from build123d import *

# Parameters (mm, degrees)
SKETCH_W             = 65
SKETCH_H             = 30
SKETCH_R             = 7.6
PAD_DEPTH            = 22.5
SKETCH001_R          = 1.6
POCKET_DEPTH         = 12.001
POCKET_DEPTH_BACK    = -18.001
POCKET001_DEPTH      = 7
POCKET002_DEPTH      = 7
SKETCH004_R          = 5.1
POCKET003_DEPTH      = 8.5
SKETCH005_R          = 1.6
POCKET004_DEPTH      = 22.501
POCKET004_DEPTH_BACK = -22.501


with BuildPart() as part:
    # Sketch → Pad (new body, symmetric)
    with BuildSketch(Plane.XZ):
        with Locations((0, 3)):
            Rectangle(SKETCH_W, SKETCH_H)
        with Locations((-22.5, 0)):
            Circle(SKETCH_R, mode=Mode.SUBTRACT)
        with Locations((22.5, 0)):
            Circle(SKETCH_R, mode=Mode.SUBTRACT)
    extrude(amount=PAD_DEPTH, both=True)

    # Sketch001 → Pocket (cut, two sides)
    with BuildSketch(Plane.XY) as pocket_sk:
        with Locations((-12.5, 17.5)):
            Circle(SKETCH001_R)
        with Locations((12.5, 17.5)):
            Circle(SKETCH001_R)
        Circle(SKETCH001_R)
        with Locations((-12.5, -17.5)):
            Circle(SKETCH001_R)
        with Locations((12.5, -17.5)):
            Circle(SKETCH001_R)
        with Locations((0, 17.5)):
            Circle(SKETCH001_R)
        with Locations((0, -17.5)):
            Circle(SKETCH001_R)
    extrude(amount=-POCKET_DEPTH, mode=Mode.SUBTRACT)
    extrude(pocket_sk.sketch, amount=-POCKET_DEPTH_BACK, mode=Mode.SUBTRACT)

    # Sketch002 (on DatumPlane) → Pocket001 (cut)
    with BuildSketch(Plane.YZ.offset(2)):
        with BuildLine():
            ThreePointArc((-7, -1.25), (-3.464466, 0.214466), (-2, 3.75))
            Line((-2, 18), (-2, 3.75))
            Line((-14, 18), (-2, 18))
            Line((-14, 1.25), (-14, 18))
            Line((-22.5, 1.25), (-14, 1.25))
            Line((-22.5, -1.25), (-22.5, 1.25))
            Line((-7, -1.25), (-22.5, -1.25))
        make_face()
        with BuildLine():
            ThreePointArc((2, 3.75), (3.464466, 0.214466), (7, -1.25))
            Line((22.5, -1.25), (7, -1.25))
            Line((22.5, 1.25), (22.5, -1.25))
            Line((14, 1.25), (22.5, 1.25))
            Line((14, 18), (14, 1.25))
            Line((2, 18), (14, 18))
            Line((2, 3.75), (2, 18))
        make_face()
    extrude(amount=POCKET001_DEPTH, mode=Mode.SUBTRACT)

    # Sketch003 (on DatumPlane) → Pocket002 (cut)
    with BuildSketch(Plane.YZ.offset(-2)):
        with BuildLine():
            Line((-7, -1.25), (-22.5, -1.25))
            Line((-22.5, -1.25), (-22.5, 1.25))
            Line((-22.5, 1.25), (-14, 1.25))
            Line((-14, 1.25), (-14, 18))
            Line((-14, 18), (-2, 18))
            Line((-2, 18), (-2, 3.75))
            ThreePointArc((-7, -1.25), (-3.464466, 0.214466), (-2, 3.75))
        make_face()
        with BuildLine():
            Line((2, 3.75), (2, 18))
            Line((2, 18), (14, 18))
            Line((14, 18), (14, 1.25))
            Line((14, 1.25), (22.5, 1.25))
            Line((22.5, 1.25), (22.5, -1.25))
            Line((22.5, -1.25), (7, -1.25))
            ThreePointArc((2, 3.75), (3.464466, 0.214466), (7, -1.25))
        make_face()
    extrude(amount=-POCKET002_DEPTH, mode=Mode.SUBTRACT)

    # Sketch004 (on DatumPlane) → Pocket003 (cut)
    with BuildSketch(Plane.XY.offset(-11)):
        with Locations((-7.4, 0)):
            Circle(SKETCH004_R)
        with Locations((7.4, 0)):
            Circle(SKETCH004_R)
    extrude(amount=POCKET003_DEPTH, mode=Mode.SUBTRACT)

    # Sketch005 → Pocket004 (cut, two sides)
    with BuildSketch(Plane.XZ) as pocket004_sk:
        with Locations((-5.5, 9.625)):
            Circle(SKETCH005_R)
        with Locations((5.5, 9.625)):
            Circle(SKETCH005_R)
    extrude(amount=-POCKET004_DEPTH, mode=Mode.SUBTRACT)
    extrude(pocket004_sk.sketch, amount=-POCKET004_DEPTH_BACK, mode=Mode.SUBTRACT)


solid = part.part
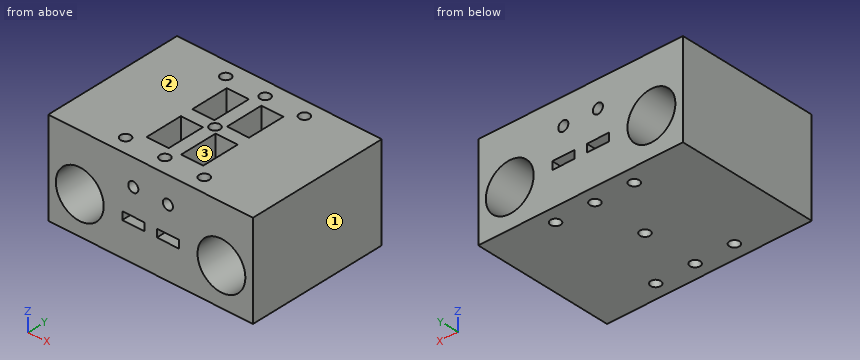
For this review, take the finished solid that the model builds, in its own axes (mm). Face numbers are marked on the shaded views. Round coordinates to 2 decimals unless told otherwise and drop trailing zeros. Write each loop counter-clockwise with the first axis right and the second up, starting at its lowest first coordinate (ties: lowest second). Pieces come first, ordered by that corner, then holes. Notation, with made-up numbers: M 58,-28.5 L 113,-28.5 A27 ccw 113,-6.5 Z; hole C 24.25,13.25 d10. An arc over 180 degrees is marked long. Write item = value, one per line. Start each with the question number.
(1) We need section C-C (x = -24). Give the boundary of the cut face in (y, z).
(2) For line 1 along X through (y, z) = (13, 14.5); line 2 along Y through (x, z) = (-12.5, 4.25); line 3 along X through (y, z) = (21.5, 0.75), list the stretches that pass through material, from the lowest coordinate up.
(3) We need section B-B (x = -5.5). Give the number of separate pieces and of enclosed holes in the cut face, then the cut area to 3 significant figures.
(4) The part is to be moulded in two halves that separate along X. For the marked faces 1, 2 and 3, say which applies: +X half, -X half, draft (parallel to the pull), parting line (faces both ways), or undercut.
(5) We need section A-A (y = -12). Give the boundary of the cut face in (x, z).
(6) Clearance check with a flat-ended pin moving along its axis: pin 1 Ø2.5 at (x, z) = (5.5, 9.625) entering from -Y. State where the tip first meets the part, or that it passes through.
Results found:
q1.outline = M -22.5,-12 L 22.5,-12 L 22.5,-7.45 L -22.5,-7.45 Z; M -22.5,7.45 L 22.5,7.45 L 22.5,18 L -22.5,18 Z
q2.line_1 = -32.5 to -9, -2 to 2, 9 to 32.5
q2.line_2 = -22.5 to -19.1, -15.9 to 15.9, 19.1 to 22.5
q2.line_3 = -32.5 to -30.06, -14.94 to -9, -2 to 2, 9 to 14.94, 30.06 to 32.5
q3.separate_pieces = 6
q3.enclosed_holes = 1
q3.area = 709 mm²
q4.face_1 = +X half
q4.face_2 = draft
q4.face_3 = undercut
q5.outline = M -32.5,-12 L 32.5,-12 L 32.5,18 L 9,18 L 9,-1.25 L 2,-1.25 L 2,18 L -2,18 L -2,-1.25 L -9,-1.25 L -9,18 L -32.5,18 Z; hole C -22.5,0 d15.2; hole C 22.5,0 d15.2
q6.pin_1 = through
